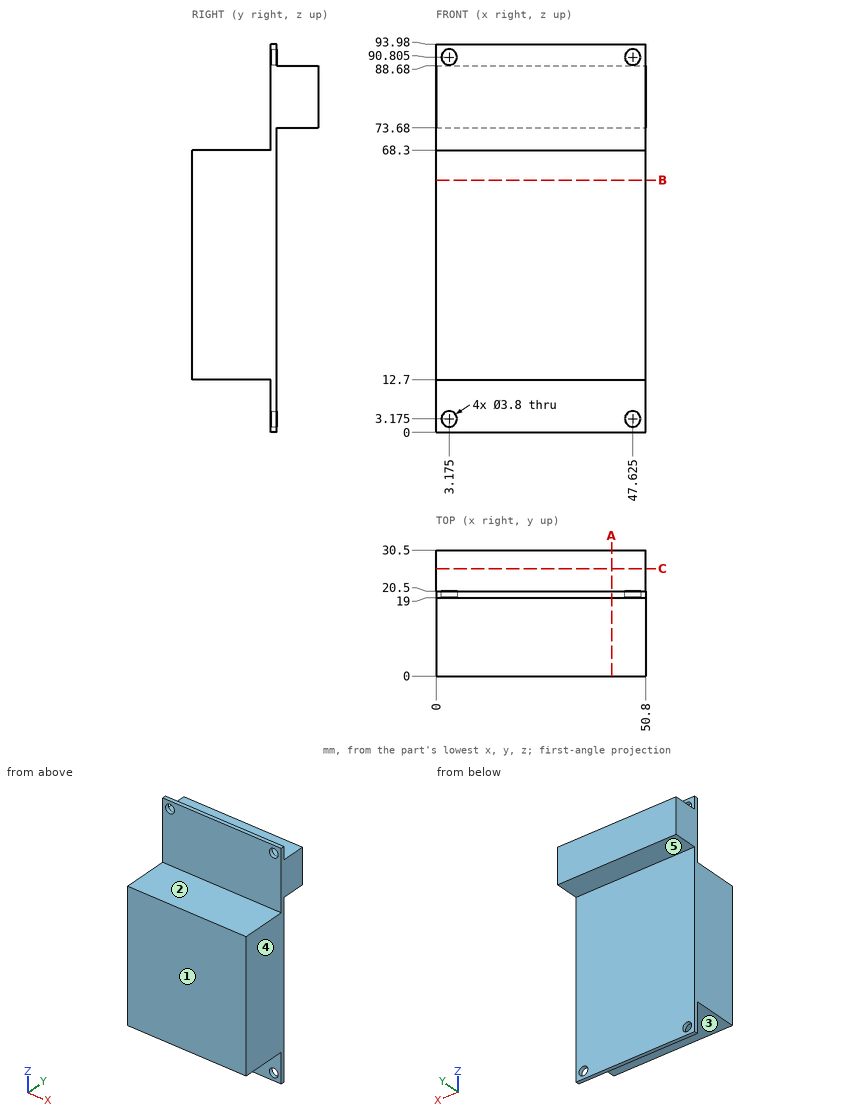
Job drawing, mm, ordinate dimensions from the low corner. One solid piece. A direction names the side the tool comes from. Give positions to 0.01 mm unless a question says otherwise; leave off trailing zeros. Write each loop counter-clockwise with the first axis right and the second up, starting at its lowest first coordinate (ties: lowest second). Pieces come first, ordered by that corner, then holes. Notation, with made-up numbers: (81.25, 75.25) - (90.25, 75.25) arc R9 cw to (90.25, 83.25) - close; hole circle Ø1 at (22, -5.75). An arc over 180 degrees is marked (long way). Answer as CSV lines item,"result".
1. Pin check, flat tips, straight feed: pin 1 (5 mm diameter, centred on x = 3.175, z = 90.805, fed in from -Y); pin 2 (2 mm diameter, centred on x = 7, y = 7, fed in from -Z); pin 3 (5.5 mm diameter, centred on x = 17, y = 12, fed in from +Z). Stop position of each tip, or through.
Responses:
pin 1,"stops at y = 19"
pin 2,"stops at z = 12.7"
pin 3,"stops at z = 68.3"
2. Drill centre lines: L1, parallel to Y at x = 16.5, z = 17; L2, parallel to Z at x = 4, y = 11; L3, parallel to Z at x = 13.5, y = 27. Where is each one in solid material? Low to high. Write a range as [from, to].
Responses:
L1,"y = [0, 20.5]"
L2,"z = [12.7, 68.3]"
L3,"z = [73.68, 88.68]"
3. Band-saw the part on C-C (y = 26). Write the cut outline in (x, z).
Responses:
outline,"(0, 73.68) - (50.8, 73.68) - (50.8, 88.68) - (0, 88.68) - close"
4. Band-saw the part on B-B (z = 61). Write the cut outline in (x, y).
Responses:
outline,"(0, 0) - (50.8, 0) - (50.8, 20.5) - (0, 20.5) - close"
5. Band-saw the part on A-A (x = 42.5). Write the cut outline in (y, z), and give its area (3 significant figures).
Responses:
outline,"(0, 12.7) - (19, 12.7) - (19, 0) - (20.5, 0) - (20.5, 73.68) - (30.5, 73.68) - (30.5, 88.68) - (20.5, 88.68) - (20.5, 93.98) - (19, 93.98) - (19, 68.3) - (0, 68.3) - close"
area,"1,350 mm2"
6. 3-axis set-ups, long thin cutter, end or side, ignore diameter. For the marked faces 1, 2, 3, 4 and 5: which of +Z, -Z, +X, -X, +Y, -Y reach the whole face in a straight line?
Responses:
face 1,"+Z, -Z, +X, -X, -Y"
face 2,"+Z, +X, -X, -Y"
face 3,"-Z, +X, -X, -Y"
face 4,"+Z, -Z, +X, +Y, -Y"
face 5,"-Z, +X, -X, +Y"
